Verification items for this drawing (mm, ordinates from the low corner). Round coordinates to 2 decimals unless told otherwise and drop trailing zeros. Order: outer loops, then holes, each group sorted by start corner. A loop starts at its lowest first (then second) coordinate and runs counter-clockwise, first axis right, second up.
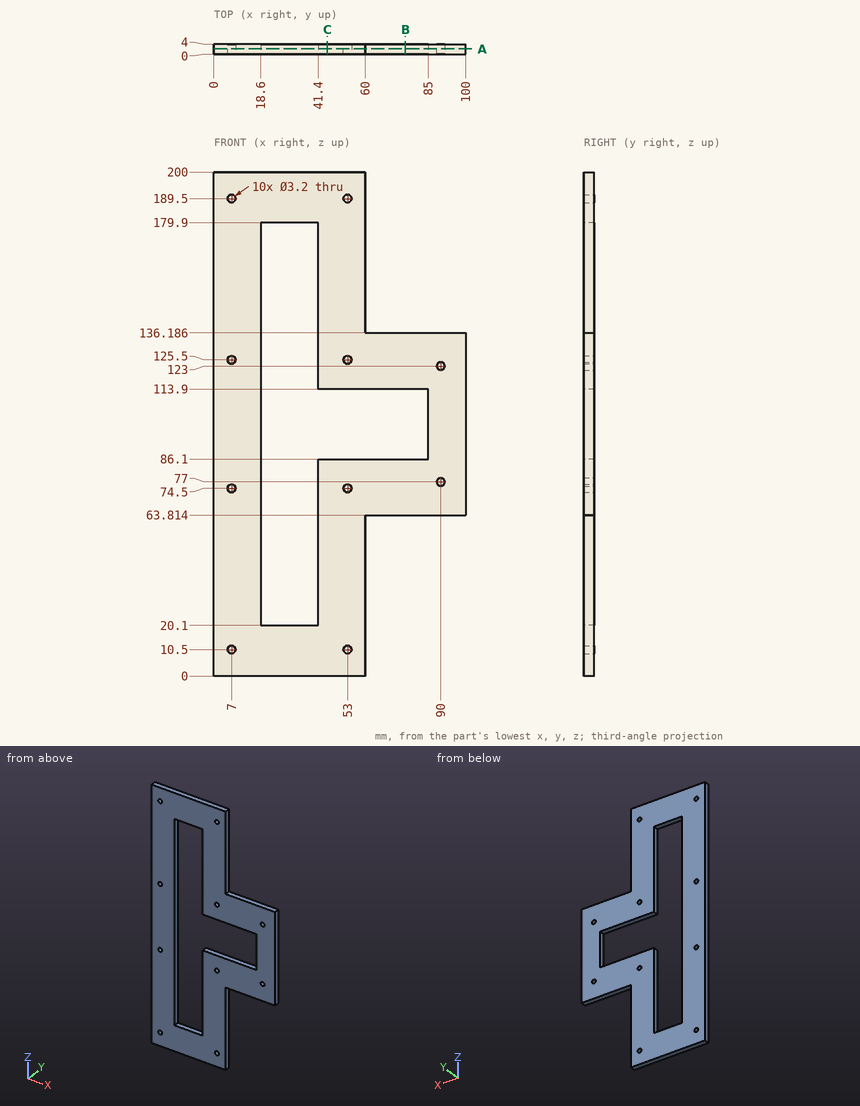
Item 1: Sectioned sample at C-C (x = 45). Record the cut outline in (y, z).
Answer:
outline: (0, 0) - (4, 0) - (4, 86.1) - (0, 86.1) - close; (0, 113.9) - (4, 113.9) - (4, 200) - (0, 200) - close
Item 2: Sectioned sample at B-B (x = 76). Record the cut outline in (y, z), and give its area (3 significant figures).
Answer:
outline: (0, 63.81) - (4, 63.81) - (4, 86.1) - (0, 86.1) - close; (0, 113.9) - (4, 113.9) - (4, 136.19) - (0, 136.19) - close
area: 178 mm2
Item 3: Sectioned sample at A-A (y = 2.1). State how many separate pieces and enclosed holes the cut face has, and give its area (3 significant figures).
Answer:
separate pieces: 1
enclosed holes: 11
area: 9,960 mm2
Item 4: Go/stop test with flat-tipped pins: P1, Ø2, axis at x = 37, y = 2.5, coming from the -Z side; P2, Ø3, axis at x = 7, z = 125.5, coming from the -Y side; P3, Ø2, axis at y = 1.5, z = 47.5, coming from the +X side; P4, Ø2, axis at x = 70.5, y = 1.5, coming from the +Z side. Record where each tip stops, or that it passes through.
Answer:
P1: stops at z = 0
P2: passes through
P3: stops at x = 60
P4: stops at z = 136.19
Item 5: Scan lines: line 1 along Z through (x, y) = (53, 3.1); line 2 along Z through (x, y) = (7, 0.8); line 3 along X through (y, z) = (1.55, 125.5). Record each from-to range of solid material in increasing order.
Answer:
line 1: z = 0 to 8.9, 12.1 to 72.9, 76.1 to 86.1, 113.9 to 123.9, 127.1 to 187.9, 191.1 to 200
line 2: z = 0 to 8.9, 12.1 to 72.9, 76.1 to 123.9, 127.1 to 187.9, 191.1 to 200
line 3: x = 0 to 5.4, 8.6 to 18.6, 41.4 to 51.4, 54.6 to 100
